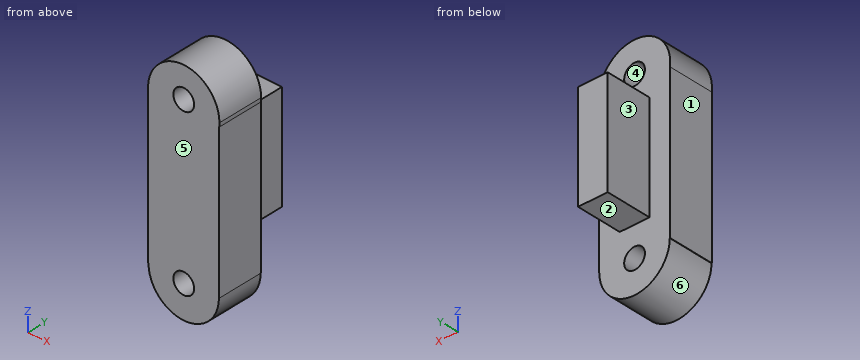
```python
from build123d import *

# Parameters (mm, degrees)
F1_DEPTH = 25.4
F2_R     = 5.715
F3_DEPTH = 25.4
F4_W     = 16.3346650079
F4_H     = 58.4679208696
F5_DEPTH = 25.4


with BuildPart() as f1:
    # F0 (on Front) → F1 (new body)
    with BuildSketch(Plane.XZ):
        with BuildLine():
            Line((-19.5532236248, 40.6393535502), (-19.5532236248, 42.7938178182))
            Line((-19.5532236248, 42.7938178182), (19.5532236248, 42.7938178182))
            Line((19.5532236248, 42.7938178182), (19.5532236248, 40.6393535502))
            ThreePointArc((19.5532236248, 40.6393535502), (19.6419535806, 41.7149619699), (19.6715599383, 42.7938178182))
            ThreePointArc((19.6715599383, 42.7938178182), (-1.0788558483, 62.4357713988), (-19.5532236248, 40.6393535502))
        make_face()
        with BuildLine():
            Line((19.5532236248, 42.7938178182), (-19.5532236248, 42.7938178182))
            Line((-19.5532236248, 42.7938178182), (-19.5532236248, 40.6393535502))
            ThreePointArc((-19.5532236248, 40.6393535502), (0, 23.1222578799), (19.5532236248, 40.6393535502))
            Line((19.5532236248, 40.6393535502), (19.5532236248, 42.7938178182))
        make_face()
        with BuildLine():
            ThreePointArc((19.5532236248, 40.6393535502), (0, 23.1222578799), (-19.5532236248, 40.6393535502))
            Line((-19.5532236248, 40.6393535502), (-19.5532236248, -42.7938178182))
            Line((-19.5532236248, -42.7938178182), (-19.4028248978, -42.7938178182))
            ThreePointArc((-19.4028248978, -42.7938178182), (0, -23.3909929204), (19.4028248978, -42.7938178182))
            Line((19.4028248978, -42.7938178182), (19.5532236248, -42.7938178182))
            Line((19.5532236248, -42.7938178182), (19.5532236248, 40.6393535502))
        make_face()
        with BuildLine():
            ThreePointArc((19.4028248978, -42.7938178182), (0, -23.3909929204), (-19.4028248978, -42.7938178182))
            Line((-19.4028248978, -42.7938178182), (19.4028248978, -42.7938178182))
        make_face()
        with BuildLine():
            Line((19.4028248978, -42.7938178182), (-19.4028248978, -42.7938178182))
            ThreePointArc((-19.4028248978, -42.7938178182), (0, -62.196642716), (19.4028248978, -42.7938178182))
        make_face()
    extrude(amount=F1_DEPTH)

    # F2 (on Front) → F3 (cut)
    with BuildSketch(Plane.XZ):
        with Locations((0, 45.5469058133)):
            Circle(F2_R)
        with Locations((0, -44.1561616667)):
            Circle(F2_R)
    extrude(amount=F3_DEPTH, mode=Mode.SUBTRACT)

    # F4 (on Front) → F5 (join)
    with BuildSketch(Plane.XZ):
        with Locations((-0.0131181441, 1.4724824578)):
            Rectangle(F4_W, F4_H)
    extrude(amount=-F5_DEPTH)


solid = f1.part
```
Design review of the part built by this model. Coordinates are the model's own, in mm. Face numbers are marked on the shaded views. A direction names the side the tool comes from. Coordinates: 2 decimals unless noted, no trailing zeros. Order: outer loops, then holes, each group sorted by start corner. A loop starts at its lowest first (then second) coordinate and runs counter-clockwise, first axis right, second up.
1) Mouldability with a two-part tool opening along Z and no side actions: class the marked faces 4, 5 and 6 as +Z half, -Z half, draft (parallel to the pull), parting line (faces both ways), or undercut.
2) Take a section at A-A, the plane x = 0. Give the boundary of the cut face in (y, z).
3) Take a section at B-B, the plane z = -14. Give the boundary of the cut face in (x, y).
4) Clearance check with flat-ended pins moving along their axes: pin 1 (5 mm diameter, centred on x = -12, y = -16.5, fed in from +Z); pin 2 (20.5 mm diameter, centred on y = -13, z = -18.5, fed in from -X); pin 3 (13 mm diameter, centred on x = 3, y = 17.5, fed in from +Z). State where each tip first meets the part, or that it passes through.
5) Take a section at D-D, the plane x = 7. Give the boundary of the cut face in (y, z).
6) Wall thickness on line 1 along Z through (x, y) = (0, -4); line 2 along Z through (x, y) = (1, -23); line 3 along Y through (x, z) = (5, 41.5): over which ranges is each line inside the solid? List them lowest first.
7) For the marked faces 1, 2 and 3, list the 3-axis set-ups (+Z, -Z, +X, -X, +Y, -Y) from which the entire face can be reached by the end or side of a thin tool; tool diameter is ignored.
8) Take a section at C-C, the plane y = 12. Give the boundary of the cut face in (x, z).
Returned:
1. face 4: undercut
1. face 5: draft
1. face 6: -Z half
2. outline: (-25.4, -62.2) - (0, -62.2) - (0, -49.87) - (-25.4, -49.87) - close; (-25.4, -38.44) - (0, -38.44) - (0, -27.76) - (25.4, -27.76) - (25.4, 30.71) - (0, 30.71) - (0, 39.83) - (-25.4, 39.83) - close; (-25.4, 51.26) - (0, 51.26) - (0, 62.47) - (-25.4, 62.47) - close
3. outline: (-19.55, -25.4) - (19.55, -25.4) - (19.55, 0) - (8.15, 0) - (8.15, 25.4) - (-8.18, 25.4) - (-8.18, 0) - (-19.55, 0) - close
4. pin 1: stops at z = 60.02
4. pin 2: stops at x = -19.55
4. pin 3: stops at z = 30.71
5. outline: (-25.4, -60.89) - (0, -60.89) - (0, -27.76) - (25.4, -27.76) - (25.4, 30.71) - (0, 30.71) - (0, 61.18) - (-25.4, 61.18) - close
6. line 1: z = -62.2 to -49.87, -38.44 to 39.83, 51.26 to 62.47
6. line 2: z = -62.17 to -49.78, -38.53 to 39.92, 51.17 to 62.44
6. line 3: y = -25.4 to 0
7. face 1: -Z, -X, +Y, -Y
7. face 2: -Z, +X, -X, +Y
7. face 3: +Z, -Z, -X, +Y
8. outline: (-8.18, -27.76) - (8.15, -27.76) - (8.15, 30.71) - (-8.18, 30.71) - close
